Job drawing, mm, ordinate dimensions from the low corner. One solid piece. A direction names the side the tool comes from. Give positions to 0.01 mm unless a question says otherwise; leave off trailing zeros. Order: outer loops, then holes, each group sorted by start corner. A loop starts at its lowest first (then second) coordinate and runs counter-clockwise, first axis right, second up. Notation, with made-up numbers: (-39, 24.5) - (17, 24.5) arc R20 ccw to (17, 29.5) - close; hole circle Ø7 at (-33.5, -12.75). An arc over 180 degrees is marked (long way). One line per item, written item: value.
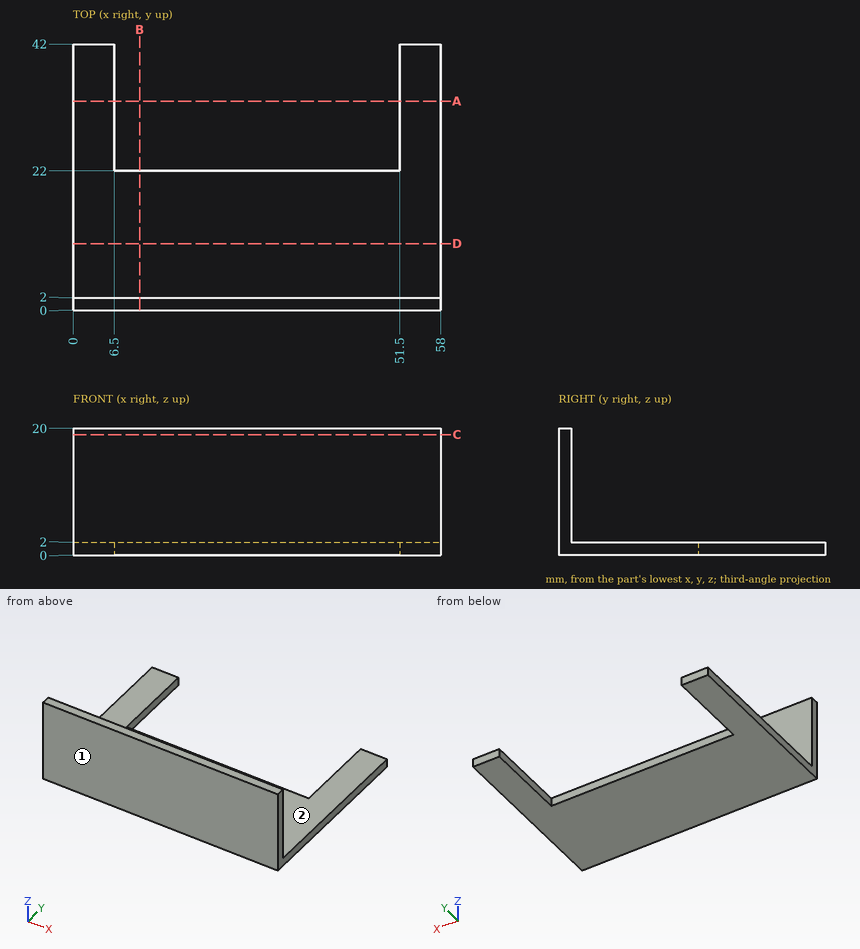
1) Slice it at A-A on y = 33. Write the cut outline in (x, z).
Answer:
outline: (0, 0) - (6.5, 0) - (6.5, 2) - (0, 2) - close; (51.5, 0) - (58, 0) - (58, 2) - (51.5, 2) - close
2) Wall check: line 1 along X through (y, z) = (40, 1.25); line 2 along Z through (x, y) = (43.5, 13.5). Give the ranges that are in metal, low to high. Write a range as [from, to].
Answer:
line 1: x = [0, 6.5], [51.5, 58]
line 2: z = [0, 2]
3) Slice it at B-B on x = 10.5. Write the cut outline in (y, z).
Answer:
outline: (0, 0) - (22, 0) - (22, 2) - (2, 2) - (2, 20) - (0, 20) - close
4) Slice it at C-C on z = 19. Write the cut outline in (x, y), then the cut area to 3 significant figures.
Answer:
outline: (0, 0) - (58, 0) - (58, 2) - (0, 2) - close
area: 116 mm2
5) Drop flat-ended pins along their axis: P1, Ø8, axis at x = 27, y = 18.5, coming from the -Z side; P2, Ø1, axis at x = 7, y = 19.5, coming from the +Z side; P3, Ø5, axis at x = 31.5, z = 2.5, coming from the +Y side. Give the stop position or say it passes through.
Answer:
P1: stops at z = 0
P2: stops at z = 2
P3: stops at y = 22
6) Which spindle directions (+Z, -Z, +X, -X, +Y, -Y) get a long thin tool onto all of the face, cutting with end or side? Do the marked faces 1 and 2. Say none if no direction does.
Answer:
face 1: +Z, -Z, +X, -X, -Y
face 2: +Z, +X, -X, +Y
